```python
from build123d import *

# Parameters (mm, degrees)
SKETCH1_R                                = 15.875
BOSS_EXTRUDE1_DEPTH                      = 6.35
SKETCH2_R                                = 6.35
CUT_EXTRUDE1_DEPTH                       = 24.3313898
F_1_16_0_0625_DIAMETER_HOLE1_D           = 1.5875
F_1_16_0_0625_DIAMETER_HOLE1_CSINK_D     = 2.8575
F_1_16_0_0625_DIAMETER_HOLE1_CSINK_ANGLE = 100
CIRPATTERN1_COUNT                        = 2
CIRPATTERN2_COUNT                        = 2


with BuildPart() as part:
    # Sketch1 → Boss-Extrude1 (new body)
    with BuildSketch(Plane(origin=(0, 0, 0), x_dir=(1, 0, 0), z_dir=(0, 1, 0))):
        with Locations(Location((0, 0, 0), (0, 0, 270))):
            Circle(SKETCH1_R)
    extrude(amount=BOSS_EXTRUDE1_DEPTH)

    # Sketch2 → Cut-Extrude1 (cut, through all)
    with BuildSketch(Plane(origin=(0, 6.35, 0), x_dir=(1, 0, 0), z_dir=(0, 1, 0))):
        with Locations(Location((0, 0, 0), (0, 0, 270))):
            Circle(SKETCH2_R)
    extrude(amount=-CUT_EXTRUDE1_DEPTH, mode=Mode.SUBTRACT)

    # 1/16 (0.0625) Diameter Hole1 (through all)
    with Locations(Plane(origin=(0, 6.35, 0), x_dir=(1, 0, 0), z_dir=(0, 1, 0))):
        with Locations((0, 11.1125)):
            f_1_16_0_0625_diameter_hole1 = CounterSinkHole(F_1_16_0_0625_DIAMETER_HOLE1_D / 2, F_1_16_0_0625_DIAMETER_HOLE1_CSINK_D / 2, counter_sink_angle=F_1_16_0_0625_DIAMETER_HOLE1_CSINK_ANGLE)

    # CirPattern1: 1/16 (0.0625) Diameter Hole1 ×2 about axis
    cirpattern1_axis = Axis((0, 0, 0), (0, 1, 0))
    for i in range(1, CIRPATTERN1_COUNT):
        add(f_1_16_0_0625_diameter_hole1.rotate(cirpattern1_axis, i * 360 / CIRPATTERN1_COUNT), mode=Mode.SUBTRACT)

    # Sketch10 → 1/16 (0.0625) Diameter Hole2 (revolve, cut)
    with BuildSketch(Plane(origin=(11.1125, 6.35, 0), x_dir=(0, 0, 1), z_dir=(1, 0, 0))):
        Polygon((0, 0), (0, 4.286933116), (0.79375, 3.81), (0.79375, 0.532828266), (1.42875, 0), align=None)
    f_1_16_0_0625_diameter_hole2 = revolve(axis=Axis((11.1125, 12.7, 0), (0, -1, 0)), mode=Mode.SUBTRACT)

    # CirPattern2: 1/16 (0.0625) Diameter Hole2 ×2 about axis
    cirpattern2_axis = Axis((0, 0, 0), (0, 1, 0))
    for i in range(1, CIRPATTERN2_COUNT):
        add(f_1_16_0_0625_diameter_hole2.rotate(cirpattern2_axis, i * 360 / CIRPATTERN2_COUNT), mode=Mode.SUBTRACT)


solid = part.part
```
Here's how the part is built. I have some questions about the finished solid (model axes, mm). A direction names the side the tool comes from. Coordinates: 2 decimals unless noted, no trailing zeros. Write each loop counter-clockwise with the first axis right and the second up, starting at its lowest first coordinate (ties: lowest second). Pieces come first, ordered by that corner, then holes. Notation, with made-up numbers: (-6, -27) -> (43, -27) arc R26 ccw to (43, 11) -> close; hole circle Ø6 at (12, -27.75). An arc over 180 degrees is marked (long way). Use a Markdown table: item, result. Add a question column.
(1) We'd pull the mould along Z, two halves only. Please class faces 1 (the flat face through (-7, 6.35, 0)), 2 (the cylindrical face through (-15.497, 3.131, -3.441)), 3 (the cylindrical face through (10.326, 4.202, -0.103)): +Z half, -Z half, draft (parallel to the pull), parting line (faces both ways), or undercut.
(2) For faces 4 (the cylindrical face through (0.4, 2.9, 11.8)), 5 (the cylindrical face through (-10.326, 4.202, 0.103)), which set-ups out of +Z, -Z, +X, -X, +Y, -Y let a thin tool reach every point of the face, with its end or its side?
(3) If we section it at A-A, the plane x = 0: Write out the boundary of the cut face in (y, z) (3 decimals).
(4) If we section it at B-B, the plane z = 4: Write out the boundary of the cut face in (x, y).
(5) If we section it at C-C, the plane y = 3.5: State how many separate pieces and enclosed holes the cut face has, and give its area (3 significant figures).
(6) I'm going to push flat-ended pins straight in: P1, Ø2, axis at y = 1, z = 6, coming from the -X side; P2, Ø2.5, axis at x = 11.11, z = 0, coming from the +Y side; P3, Ø1, axis at x = 7.5, y = 5, coming from the +Z side; P4, Ø1, axis at x = 0, z = 11.11, coming from the -Y side. Where does each tip first touch, or does it pass through?
(7) Please list where these lines run through material, in increasing order: line 1 (X direction, y = 3.95, z = 0) (3 decimals); line 2 (Z direction, x = 2.5, y = 3.5); line 3 (Z direction, x = 5, y = 1).
Outcome:
| question | item | result |
|---|---|---|
| 1 | face 1 | draft |
| 1 | face 2 | parting line |
| 1 | face 3 | undercut |
| 2 | face 4 | +Y, -Y |
| 2 | face 5 | +Y |
| 3 | outline | (0, -15.875) -> (6.35, -15.875) -> (6.35, -12.541) -> (5.817, -11.906) -> (0, -11.906) -> close; (0, -10.319) -> (5.817, -10.319) -> (6.35, -9.684) -> (6.35, -6.35) -> (0, -6.35) -> close; (0, 6.35) -> (6.35, 6.35) -> (6.35, 9.684) -> (5.817, 10.319) -> (0, 10.319) -> close; (0, 11.906) -> (5.817, 11.906) -> (6.35, 12.541) -> (6.35, 15.875) -> (0, 15.875) -> close |
| 4 | outline | (-15.36, 0) -> (-4.93, 0) -> (-4.93, 6.35) -> (-15.36, 6.35) -> close; (4.93, 0) -> (15.36, 0) -> (15.36, 6.35) -> (4.93, 6.35) -> close |
| 5 | separate pieces | 1 |
| 5 | enclosed holes | 5 |
| 5 | area | 657 mm^2 |
| 6 | P1 | stops at x = -15.07 |
| 6 | P2 | stops at y = 6.2 |
| 6 | P3 | stops at z = 14.25 |
| 6 | P4 | passes through |
| 7 | line 1 | x = -15.875 to -11.906, -10.319 to -6.35, 6.35 to 10.319, 11.906 to 15.875 |
| 7 | line 2 | z = -15.68 to -5.84, 5.84 to 15.68 |
| 7 | line 3 | z = -15.07 to -3.91, 3.91 to 15.07 |
